from build123d import *

# Parameters (mm, degrees)
F0_R     = 30.095245
F1_DEPTH = 6
F2_R     = 25.269078
F3_DEPTH = 15
F4_R     = 6.785687
F5_DEPTH = 14
F6_R     = 1
F7_R     = 1
F8_SIZE  = 1


with BuildPart() as f1:
    # F0 (on Top) → F1 (new body)
    with BuildSketch(Plane.XY):
        Circle(F0_R)
    extrude(amount=F1_DEPTH)

    # F2 (on face) → F3 (join)
    with BuildSketch(Plane.XY.offset(6)):
        Circle(F2_R)
    extrude(amount=F3_DEPTH)

    # F4 (on face) → F5 (cut)
    with BuildSketch(Plane.XY.offset(21)):
        Circle(F4_R)
    extrude(amount=-F5_DEPTH, mode=Mode.SUBTRACT)

    # F6
    f6_edges = [f1.edges().sort_by_distance(p)[0] for p in [
        (-30.095245, 0, 6),
    ]]
    fillet(f6_edges, radius=F6_R)

    # F7
    f7_edges = [f1.edges().sort_by_distance(p)[0] for p in [
        (-30.095245, 0, 0),
    ]]
    fillet(f7_edges, radius=F7_R)

    # F8
    f8_edges = [f1.edges().sort_by_distance(p)[0] for p in [
        (-25.269078, 0, 21),
    ]]
    chamfer(f8_edges, length=F8_SIZE)


solid = f1.part
Could you check a few things on this model? Use its own coordinates, in mm. A direction names the side the tool comes from. Give positions to 0.01 mm unless a question says otherwise; leave off trailing zeros. Order: outer loops, then holes, each group sorted by start corner. A loop starts at its lowest first (then second) coordinate and runs counter-clockwise, first axis right, second up. Notation, with made-up numbers: (11.25, 36.25) - (42.25, 36.25) arc R31 cw to (42.25, 64.25) - close; hole circle Ø1 at (0.25, 6.25). An arc over 180 degrees is marked (long way). One line per question, with ' | ' between items. Start each with the question number.
Item 1: I want a section at D-D on z = 12.75. Write out the boundary of the cut face in (x, y), then the cut area to 3 significant figures.
Item 2: I need wall thicknesses on probe 1 along Y at (x, z) = (0, 15.25); probe 2 along Z at (x, y) = (20, 18.5); probe 3 along X at (y, z) = (-5, 16.25). Which ranges of each line are inside material? Lowest first, please. Write a range as [from, to].
Item 3: Thinking about a two-plate mould opening in X: for faces 1 (the flat face through (-9, 24, 6)), 2 (the flat face through (0, 0, 7)), 3 (the cylindrical face through (6.47, 2.04, 14.1)), 4 (the cylindrical face through (-3.92, 29.84, 2.97)), which applies, pulls with the +X half, pulls with the -X half, needs draft (parallel to the pull), parting line crosses it, or undercut?
Item 4: I want a section at A-A on x = 0. Write out the boundary of the cut face in (y, z), then the cut area to 3 significant figures.
Item 5: For faces 5 (the flat face through (0, 0, 0)), 6 (the cylindrical face through (-3.29, 25.054, 12.902)), which set-ups out of +Z, -Z, +X, -X, +Y, -Y let a thin tool reach every point of the face, with its end or its side?
Item 6: I'm going to push flat-ended pins straight in: pin 1 Ø1.5 at (x, z) = (-16.5, 8.5) entering from +Y; pin 2 Ø2 at (x, z) = (22.5, 11) entering from +Y; pin 3 Ø1.5 at (x, z) = (8, 8) entering from +Y. Where does each tip first touch, or does it pass through?
Item 7: I want a section at C-C on z = 2. Write out the boundary of the cut face in (x, y), then the cut area to 3 significant figures.
Verdict:
1) outline: circle Ø50.54 at (0, 0); hole circle Ø13.57 at (0, 0) | area: 1,860 mm^2
2) probe 1: [-25.27, -6.79], [6.79, 25.27] | probe 2: [0, 6] | probe 3: [-24.77, -4.59], [4.59, 24.77]
3) face 1: needs draft | face 2: undercut | face 3: undercut | face 4: parting line crosses it
4) outline: (-30.1, 1) arc R1 ccw to (-29.1, 0) - (29.1, 0) arc R1 ccw to (30.1, 1) - (30.1, 5) arc R1 ccw to (29.1, 6) - (25.27, 6) - (25.27, 20) - (24.27, 21) - (6.79, 21) - (6.79, 7) - (-6.79, 7) - (-6.79, 21) - (-24.27, 21) - (-25.27, 20) - (-25.27, 6) - (-29.1, 6) arc R1 ccw to (-30.1, 5) - close | area: 927 mm^2
5) face 5: -Z, +X, -X, +Y, -Y | face 6: +Z
6) pin 1: y = 19.76 | pin 2: y = 13.28 | pin 3: y = 24.21
7) outline: circle Ø60.19 at (0, 0) | area: 2,850 mm^2
